Design review of the part shown in the three views and the two pictorial views. Dimensions are in mm from the part's minimum x, y and z. A direction names the side the tool comes from. Give positions to 0.01 mm unless a question says otherwise; leave off trailing zeros. Loops run counter-clockwise (first coordinate to the right, second up) from the corner with the lowest first, then second, coordinate; pieces in that order, holes last. Notation, with made-up numbers: (5, 45) - (20, 45) arc R9 ccw to (20, 52) - close; hole circle Ø3 at (-18.75, 85). An arc over 180 degrees is marked (long way). Return JSON: item names as keys, results as strings. Group by question number.
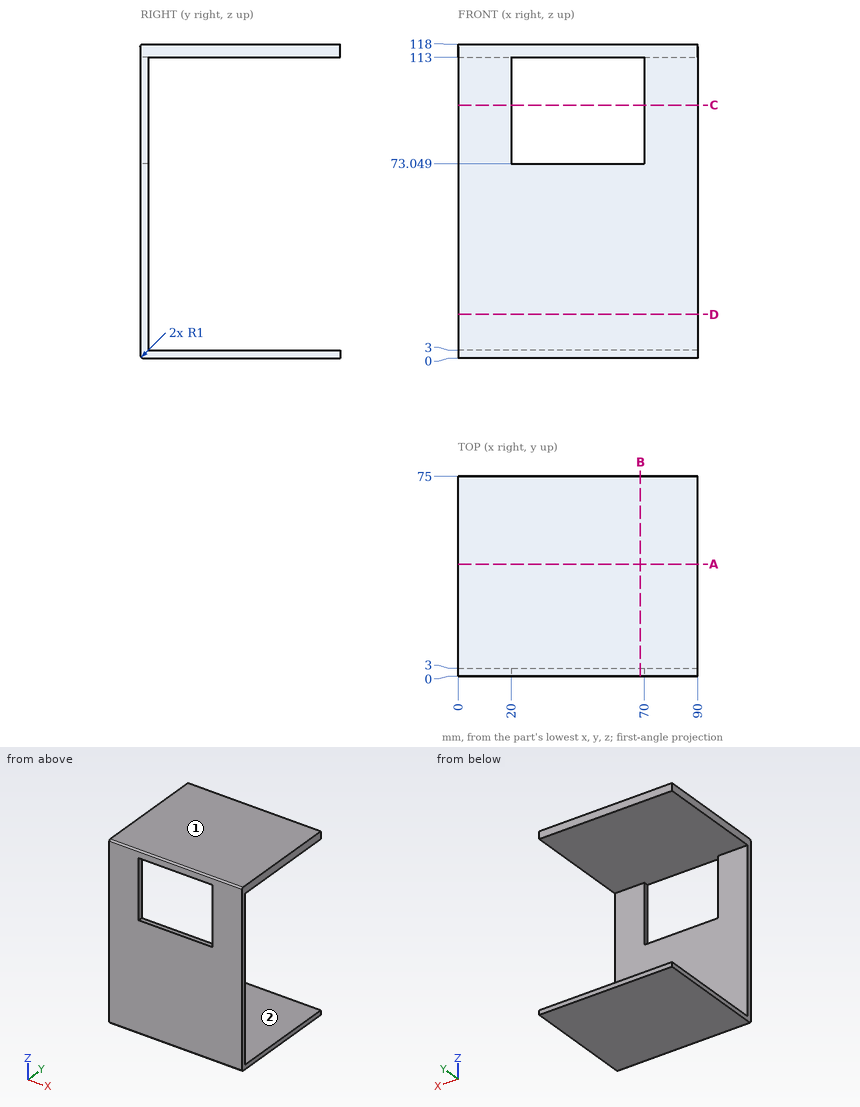
Item 1: For L1, parallel to Z at x = 57.5, y = 36.5; L2, parallel to Y at x = 11, z = 18, list the stretches that pass through material, from the lowest coordinate up. Write a range as from..to.
Item 2: Take a section at B-B (x = 68.5). State the section outline as (y, z) points.
Item 3: Tool access review of the marked faces 1 and 2: name each direction out of +Z, -Z, +X, -X, +Y, -Y from which nothing blocks a thin tool from reaching the whole face with its end or side.
Item 4: Take a section at A-A (y = 42). State the section outline as (x, z) points, then the cut area to 3 significant figures.
Item 5: Take a section at C-C (z = 95). State the section outline as (x, y) points.
Item 6: Take a section at D-D (z = 16.5). State the section outline as (x, y) points.
Check sheet entries:
{
 "1": {"L1": "z = 0..3, 113..118", "L2": "y = 0..3"},
 "2": {"outline": "(0, 1) arc R1 ccw to (1, 0) - (75, 0) - (75, 3) - (3, 3) - (3, 73.05) - (0, 73.05) - close; (0, 113) - (75, 113) - (75, 118) - (1, 118) arc R1 ccw to (0, 117) - close"},
 "3": {"face 1": "+Z, +X, -X, +Y, -Y", "face 2": "+X, -X, +Y"},
 "4": {"outline": "(0, 0) - (90, 0) - (90, 3) - (0, 3) - close; (0, 113) - (90, 113) - (90, 118) - (0, 118) - close", "area": "720 mm^2"},
 "5": {"outline": "(0, 0) - (20, 0) - (20, 3) - (0, 3) - close; (70, 0) - (90, 0) - (90, 3) - (70, 3) - close"},
 "6": {"outline": "(0, 0) - (90, 0) - (90, 3) - (0, 3) - close"}
}
